```python
from build123d import *

# Parameters (mm, degrees)
F1_DEPTH = 63.5
F0_W     = 25.4
F0_H     = 19.05
F2_DEPTH = 25.4
F3_DEPTH = 7.9375


with BuildPart() as f1:
    # F0 (on Front) → F1 (new body, symmetric)
    with BuildSketch(Plane.XZ):
        Polygon((41.275, -9.525), (41.275, 9.525), (22.225, 9.525), (-41.275, 9.525), (-41.275, -9.525), align=None)
    extrude(amount=F1_DEPTH, both=True)

    # F0 (on Front) → F2 (join, symmetric)
    with BuildSketch(Plane.XZ):
        with BuildLine():
            Line((22.225, 9.525), (41.275, 9.525))
            Line((41.275, 9.525), (41.275, 27.0002))
            ThreePointArc((41.275, 27.0002), (45.9246798487, 38.2255201513), (57.15, 42.8752))
            Line((57.15, 42.8752), (60.325, 42.8752))
            Line((60.325, 42.8752), (60.325, 61.9252))
            Line((60.325, 61.9252), (57.15, 61.9252))
            add(Edge.make_bspline(
                [(55.5932773948, 61.8904886163), (56.1098349358, 61.9028294033), (56.628740299, 61.9143991352), (57.15, 61.9252)],
                knots=[110.6833080475, 110.6833080475, 110.6833080475, 110.6833080475, 111.5045361635, 111.5045361635, 111.5045361635, 111.5045361635], degree=3))
            ThreePointArc((55.5932773948, 61.8904886163), (31.9099112325, 51.1392460459), (22.225, 27.0002))
            Line((22.225, 27.0002), (22.225, 9.525))
        make_face()
        with Locations((73.025, 52.4002)):
            Rectangle(F0_W, F0_H)
    extrude(amount=F2_DEPTH, both=True)

    # F0 (on Front) → F3 (join, symmetric)
    with BuildSketch(Plane.XZ):
        with BuildLine():
            Line((-41.275, 9.525), (22.225, 9.525))
            Line((22.225, 9.525), (22.225, 27.0002))
            ThreePointArc((22.225, 27.0002), (31.9099112325, 51.1392460459), (55.5932773948, 61.8904886163))
            add(Edge.make_bspline(
                [(-41.275, 9.525), (-40.9993751312, 44.557704562), (-14.0272048052, 60.2272246577), (55.5932773948, 61.8904886163)],
                knots=[0, 0, 0, 0, 110.6833080475, 110.6833080475, 110.6833080475, 110.6833080475], degree=3))
        make_face()
    extrude(amount=F3_DEPTH, both=True)


solid = f1.part
```
Design review of the part built by this model. Coordinates are the model's own, in mm. A direction names the side the tool comes from. Coordinates: 2 decimals unless noted, no trailing zeros. Write each loop counter-clockwise with the first axis right and the second up, starting at its lowest first coordinate (ties: lowest second). Pieces come first, ordered by that corner, then holes.
1) Add section A-A (x = 72). Write out the cut boundary in (y, z).
2) Add section B-B (z = 1). Write out the cut boundary in (x, y) (3 decimals).
3) Insertion check: pin 1 (12 mm diameter, centred on x = -13.5, z = 25, fed in from -Y); pin 2 (4 mm diameter, centred on y = 19.5, z = 21, fed in from +X) (3 decimals); pin 3 (5 mm diameter, centred on y = 19.5, z = 21.5, fed in from -X) (3 decimals). Each pin has a flat end and moves straight along its axis. Give the tip position at first contact, or say it passes through.
4) Machinability: for faces 1 (the flat face through (46, 25.4, 42)), 2 (the cylindrical face through (32.17, 16.55, 51.41)), 3 (the flat face through (71, 0, 42.875)), which of the approach directions +Z, -Z, +X, -X, +Y, -Y give a long, thin tool a straight path to every point of the face, cutting with its end or side? Answer none if there is none.
5) To check wall thickness, follow L1, parallel to Z at x = 10, y = 39 (3 decimals); L2, parallel to Y at x = 13.5, z = 12.5; L3, parallel to X at y = -9, z = -5.5 (3 decimals). State the ranges of each line that lie inside material, in increasing order.
Check result:
1. outline: (-25.4, 42.88) - (25.4, 42.88) - (25.4, 61.93) - (-25.4, 61.93) - close
2. outline: (-41.275, -63.5) - (41.275, -63.5) - (41.275, 63.5) - (-41.275, 63.5) - close
3. pin 1: stops at y = -7.94
3. pin 2: stops at x = 41.275
3. pin 3: stops at x = 22.225
4. face 1: +Z, +X, -X, +Y
4. face 2: +Z, -X, +Y
4. face 3: -Z, +X, +Y, -Y
5. L1: z = -9.525 to 9.525
5. L2: y = -7.94 to 7.94
5. L3: x = -41.275 to 41.275
